Geometry: final body of the model. Coordinates: model frame, mm. A direction names the side the tool comes from. Give positions to 0.01 mm unless a question says otherwise; leave off trailing zeros. Loops run counter-clockwise (first coordinate to the right, second up) from the corner with the lowest first, then second, coordinate; pieces in that order, holes last. Notation, with made-up numbers: (69.25, 83) - (92.25, 83) arc R7 cw to (92.25, 88) - close; hole circle Ø11 at (-23.5, 72.25). An arc over 180 degrees is marked (long way). Use CSV: the item, a comma, the result in double quotes. Start each with the question number.
```python
from build123d import *

# Parameters (mm, degrees)
SKETCH1_R           = 12.7
BOSS_EXTRUDE1_DEPTH = 5
SKETCH2_R           = 6
BOSS_EXTRUDE2_DEPTH = 4.2
SKETCH3_R           = 3
CUT_EXTRUDE1_DEPTH  = 21.179692763
SKETCH6_R           = 1.158179442
CUT_EXTRUDE2_DEPTH  = 19.643497526
SKETCH7_R           = 1.5
CUT_EXTRUDE3_DEPTH  = 8.2


with BuildPart() as part:
    # Sketch1 → Boss-Extrude1 (new body)
    with BuildSketch(Plane(origin=(0, 0, 0), x_dir=(1, 0, 0), z_dir=(0, 1, 0))):
        with Locations(Location((0, 0, 0), (0, 0, 270))):
            Circle(SKETCH1_R)
    extrude(amount=BOSS_EXTRUDE1_DEPTH)

    # Sketch2 → Boss-Extrude2 (add)
    with BuildSketch(Plane(origin=(0, 5, 0), x_dir=(1, 0, 0), z_dir=(0, 1, 0))):
        with Locations(Location((0, 0, 0), (0, 0, 270))):
            Circle(SKETCH2_R)
    extrude(amount=BOSS_EXTRUDE2_DEPTH)

    # Sketch3 → Cut-Extrude1 (cut, through all)
    with BuildSketch(Plane(origin=(0, 9.2, 0), x_dir=(1, 0, 0), z_dir=(0, 1, 0))):
        with Locations(Location((0, 0, 0), (0, 0, 270))):
            Circle(SKETCH3_R)
    extrude(amount=-CUT_EXTRUDE1_DEPTH, mode=Mode.SUBTRACT)

    # Sketch6 → Cut-Extrude2 (cut, through all)
    with BuildSketch(Plane(origin=(0, 5, 0), x_dir=(1, 0, 0), z_dir=(0, 1, 0))):
        with Locations(Location((-9.5, 0, 0), (0, 0, 270))):
            Circle(SKETCH6_R)
        with Locations(Location((-4.75, 8.227241336, 0), (0, 0, 270))):
            Circle(SKETCH6_R)
        with Locations(Location((4.75, 8.227241336, 0), (0, 0, 270))):
            Circle(SKETCH6_R)
        with Locations(Location((9.5, 0, 0), (0, 0, 270))):
            Circle(SKETCH6_R)
        with Locations(Location((4.75, -8.227241336, 0), (0, 0, 270))):
            Circle(SKETCH6_R)
        with Locations(Location((-4.75, -8.227241336, 0), (0, 0, 270))):
            Circle(SKETCH6_R)
    extrude(amount=-CUT_EXTRUDE2_DEPTH, mode=Mode.SUBTRACT)

    # Sketch7 → Cut-Extrude3 (cut)
    with BuildSketch(Plane(origin=(0, 5, 0), x_dir=(-0.5000000000000102, 0, 0.8660254037844328), z_dir=(-0.8660254037844328, 0, -0.5000000000000102))):
        with Locations((0, 2.1)):
            Circle(SKETCH7_R)
    extrude(amount=-CUT_EXTRUDE3_DEPTH, mode=Mode.SUBTRACT)


solid = part.part
```
Item 1: Pin query (flat end, axial travel): pin 1 Ø1 at (y, z) = (4, -5.5) entering from -X; pin 2 Ø4 at (y, z) = (6.5, -9) entering from +X; pin 3 Ø4 at (x, y) = (-10, 5.5) entering from +Z. Return the tip coordinate at first contact, or that it passes through.
Item 2: Mould query, pull axis X, two halves, no side actions, for faces 3 (the cylindrical face through (-7.7, 2.5, -10.1)), 4 (the flat face through (-5.5, 5, -3)), 5 (the cylindrical face through (-8.35, 2.54, -0.15)). Classes: pulls with the +X half, pulls with the -X half, needs draft (parallel to the pull), parting line crosses it, or undercut.
Item 3: Section B-B (x = 0). Output: boundary loops of the cut face in (y, z), plus the area to 3 significant figures.
Item 4: Section A-A (y = 1.75). Output: boundary loops of the cut face in (x, z).
Item 5: Section C-C (z = -8). Output: boundary loops of the cut face in (x, y), plus the area to 3 significant figures.
Item 6: Section D-D (x = -10). Output: boundary loops of the cut face in (y, z).
Item 7: Ray query, probe 1 along X at (y, z) = (1, 8.25); probe 2 along Y at (x, z) = (10, -7.25); probe 3 along Z at (x, y) = (-4, 3.5). Return the intervals inside material, ascending.
Item 8: Reachability of faces 1 (the cylindrical face through (-5.857, 7.071, -1.301)), 2 (the cylindrical face through (10.65, 2.54, -0.15)) from +Z, -Z, +X, -X, +Y, -Y: full face, straight path, thin tool, end or side. Return the list, or none.
Outcome:
1,pin 1,"stops at x = -11.67"
1,pin 2,"stops at x = 10.12"
1,pin 3,"stops at z = 9.81"
2,face 3,"parting line crosses it"
2,face 4,"needs draft"
2,face 5,"undercut"
3,outline,"(0, -12.7) - (5, -12.7) - (5, -6) - (9.2, -6) - (9.2, -3) - (0, -3) - close; (0, 3) - (9.2, 3) - (9.2, 6) - (5, 6) - (5, 12.7) - (0, 12.7) - close"
3,area,"122 mm2"
4,outline,"circle Ø25.4 at (0, 0); hole circle Ø2.32 at (-9.5, 0); hole circle Ø2.32 at (-4.75, -8.23); hole circle Ø2.32 at (-4.75, 8.23); hole circle Ø6 at (0, 0); hole circle Ø2.32 at (4.75, -8.23); hole circle Ø2.32 at (4.75, 8.23); hole circle Ø2.32 at (9.5, 0)"
5,outline,"(-9.86, 0) - (-5.89, 0) - (-5.89, 5) - (-9.86, 5) - close; (-3.61, 0) - (3.61, 0) - (3.61, 5) - (-3.61, 5) - close; (5.89, 0) - (9.86, 0) - (9.86, 5) - (5.89, 5) - close"
5,area,"75.9 mm2"
6,outline,"(0, -7.83) - (5, -7.83) - (5, -1.04) - (0, -1.04) - close; (0, 1.04) - (5, 1.04) - (5, 7.83) - (0, 7.83) - close"
7,probe 1,"x = -9.66 to -5.91, -3.59 to 3.59, 5.91 to 9.66"
7,probe 2,"y = 0 to 5"
7,probe 3,"z = -12.05 to -9.11, -7.34 to 7.34, 9.11 to 12.05"
8,face 1,"+Y"
8,face 2,"+Y, -Y"
